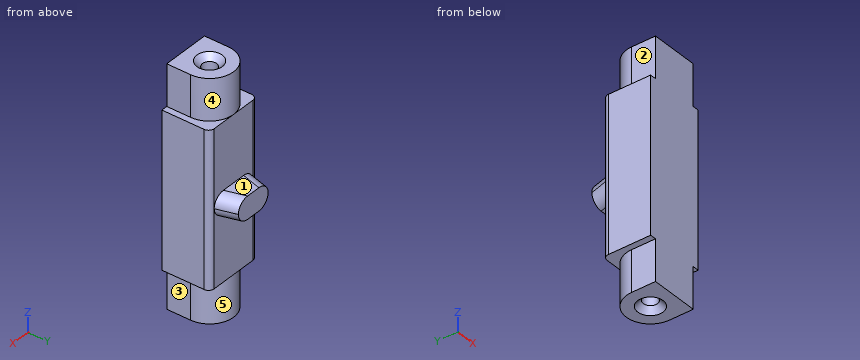
Autodesk Inventor part; units mm, degrees
ref_plane "YZ Plane" through (0, 0, 0) normal (1, 0, 0) x (0, 1, 0)
ref_plane "XZ Plane" through (0, 0, 0) normal (0, 1, 0) x (-1, 0, 0)
ref_plane "XY Plane" through (0, 0, 0) normal (0, 0, 1) x (1, 0, 0)
sketch "Sketch1" plane through (0, 0, 0) normal (0, 1, 0) x (-1, 0, 0)
  line L0 (0, 0) -> (10.7, 0)
  line L1 (10.7, 0) -> (10.7, -42)
  line L2 (10.7, -42) -> (0, -42)
  line L3 (0, -42) -> (0, 0)
  dimension "p" = 10.7
  dimension "d1" = 42
extrude "Extrusion1" add sketch "Sketch1" along normal blind 8.5
sketch "Sketch2" plane through (-10.7, 0, 0) normal (0, 0, 1) x (1, 0, 0)
  circle A0 centre (5.35, 4.25) radius 1.25
  line L0 (0, 8.5) -> (10.7, 8.5)
  line L1 (0, 0) -> (0, 8.5)
  point P0 (10.7, 0)
  dimension "d4" = 2.5
  dimension "d5" = 4.25
  dimension "d6" = 5.35
extrude "Extrusion2" cut sketch "Sketch2" against normal through all
sketch "Sketch3" plane through (-10.7, 0, 0) normal (0, 0, 1) x (1, 0, 0)
  circle A0 centre (5.35, 4.25) radius 1.25
  arc A1 (9.6, 4.25) -> (1.1, 4.25) centre (5.35, 4.25) ccw
  line L0 (10.7, 8.5) -> (0, 8.5)
  line L1 (0, 8.5) -> (10.7, 8.5)
  line L2 (10.7, 0) -> (10.7, 8.5)
  line L3 (10.7, 8.5) -> (10.7, 0)
  line L4 (0, 0) -> (10.7, 0)
  line L5 (10.7, 0) -> (0, 0)
  line L6 (0, 0) -> (0, 8.5)
  line L7 (0, 0) -> (0, 8.5)
  line L8 (10.7, 0) -> (0, 0)
  line L9 (5.35, 0) -> (1.1, 0)
  line L10 (1.1, 0) -> (1.1, 4.25)
  line L11 (5.35, 0) -> (9.6, 0)
  line L12 (9.6, 0) -> (9.6, 4.25)
  dimension "d35" = 4.25
  dimension "d36" = 4.25
  dimension "d37" = 4.25
extrude "Extrusion3" cut sketch "Sketch3" against normal blind 7.3 contours A1 L0 L2 L4 L12 | A1 L10 L4 L6 L0
sketch "Sketch4" plane through (0, 0, -42) normal (0, 0, -1) x (-1, 0, 0)
  circle A0 centre (5.35, 4.25) radius 1.25
  arc A1 (9.6, 4.25) -> (1.1, 4.25) centre (5.35, 4.25) ccw
  line L0 (0, 8.5) -> (10.7, 8.5)
  line L1 (10.7, 0) -> (0, 0)
  line L2 (0, 8.5) -> (0, 0)
  line L3 (0, 0) -> (10.7, 0)
  line L4 (10.7, 0) -> (10.7, 8.5)
  line L5 (10.7, 8.5) -> (0, 8.5)
  line L6 (1.1, 0) -> (1.1, 4.25)
  line L7 (1.1, 4.25) -> (1.1, 0)
  line L8 (9.6, 4.25) -> (9.6, 0)
  line L9 (1.1, 0) -> (9.6, 0)
  line L10 (9.6, 4.25) -> (9.6, 0)
extrude "Extrusion4" cut sketch "Sketch4" against normal blind 7.3 contours A1 L0 L4 L1 L8 | A1 L6 L1 L2 L0
sketch "Sketch5" plane through (0, 8.5, 0) normal (0, 1, 0) x (1, 0, 0)
  line L0 (-10.7, 7.3) -> (-10.7, 34.7)
  line L1 (0, 34.7) -> (0, 7.3)
  line L2 (-1, 23) -> (-9.7, 23)
  line L3 (-9.7, 19) -> (-1, 19)
  line L4 (-9.7, 19) -> (-9.7, 23)
  line L5 (-1, 19) -> (-1, 23)
  point P0 (0, 0)
  dimension "d19" = 4
  dimension "d20" = 4
  dimension "d21" = 8.7
  dimension "d22" = 1
  dimension "d23" = 19
extrude "Extrusion5" add sketch "Sketch5" along normal blind 3.5
sketch "Sketch6" plane through (-1, 8.5, -23) normal (0, 0, -1) x (-1, 0, 0)
  line L0 (8.7, 3.5) -> (0, 3.5)
  line L1 (8.7, 3.5) -> (7.7, 3.5)
  line L2 (0, 0) -> (8.7, 0)
  line L3 (7.7, 3.5) -> (8.7, 0)
  line L4 (8.7, 0) -> (8.7, 3.5)
  line L5 (0, 3.5) -> (1, 3.5)
  line L6 (1, 3.5) -> (0, 0)
  line L7 (0, 0) -> (0, 3.5)
  point P0 (-1, -8.5)
  dimension "d26" = 1
  dimension "d27" = 1
extrude "Extrusion6" cut sketch "Sketch6" against normal through all contours L4 L3 L0 | L6 L7 L0
fillet "Fillet1" radius 2 4 edges at (-1.5, 10.25, -19) (-1.5, 10.25, -23) (-9.2, 10.25, -19) (-9.2, 10.25, -23)
fillet "Fillet2" radius 1 2 edges at (0, 8.5, -21) (-10.7, 8.5, -21)
chamfer "Chamfer1" distance 1 angle 45 2 edges at (-6.6, 4.25, -42) (-6.6, 4.25, 0)
equation "\"d6\" = 0.5 * p"
properties part number "tracks_center_sod_ii"
Could you check a few things on this model? Use its own coordinates, in mm. Face numbers are marked on the shaded views. A direction names the side the tool comes from. Give positions to 0.01 mm unless a question says otherwise; leave off trailing zeros. Loops run counter-clockwise (first coordinate to the right, second up) from the corner with the lowest first, then second, coordinate; pieces in that order, holes last. Notation, with made-up numbers: (78, 40) - (124, 40) arc R30 cw to (124, 77) - close; hole circle Ø2 at (-7.75, 16). An arc over 180 degrees is marked (long way). Use one line per item in the form item = value.
1. On a 3-axis mill with a long thin cutter (end or side, diameter ignored), from which of +Z, -Z, +X, -X, +Y, -Y can I reach the whole of each face in a straight line? I mean the marked faces 1, 2, 3, 4 and 5. Say none if no direction works.
Response values:
face_1 = +Z, +X, -X, +Y
face_2 = +Z, -X, +Y, -Y
face_3 = -Z, +X, +Y, -Y
face_4 = +Z, +Y
face_5 = -Z, +Y
2. I want a section at A-A (z = -9). Please give me the cut outline in (x, y).
Response values:
outline = (-10.7, 0) - (0, 0) - (0, 7.5) arc R1 ccw to (-1, 8.5) - (-9.7, 8.5) arc R1 ccw to (-10.7, 7.5) - close; hole circle Ø2.5 at (-5.35, 4.25)
3. I need wall thicknesses on probe 1 along Y at (x, z) = (-5.35, -17.5); probe 2 along Y at (x, z) = (-4.5, -20.5); probe 3 along Z at (x, y) = (-0.75, 4.5). Which ranges of each line are inside material? Lowest first, please.
Response values:
probe_1 = 0 to 3, 5.5 to 8.5
probe_2 = 0 to 3.33, 5.17 to 12
probe_3 = -34.7 to -7.3
4. I'm going to push flat-ended pins straight in: pin 1 Ø4.5 at (x, y) = (-9, 3) entering from +Z; pin 2 Ø3 at (y, z) = (9.5, -12.5) entering from +X; pin 3 Ø2 at (y, z) = (2, -2.5) entering from -X; pin 4 Ø2 at (x, y) = (-6, 10) entering from -Z. Where does each tip first touch, or does it pass through?
Response values:
pin_1 = 0
pin_2 = -0.13
pin_3 = -9.6
pin_4 = -23
